Geometry check sheet. Reference: the model listing, model coordinates, mm. Coordinates: 2 decimals unless noted, no trailing zeros. Loops run counter-clockwise (first coordinate to the right, second up) from the corner with the lowest first, then second, coordinate; pieces in that order, holes last.
from build123d import *

# Parameters (mm, degrees)
SKETCH_1_W          = 482.6
SKETCH_1_H          = 88.1
EXTRUDE_1_DEPTH     = 4
CUT_EXTRUDE_1_DEPTH = 491.591856842
SKETCH_3_R          = 3
CUT_EXTRUDE_2_DEPTH = 491.591856842
SKETCH_4_W          = 86
SKETCH_4_H          = 55.5
CUT_EXTRUDE_3_DEPTH = 491.591856842


with BuildPart() as part:
    # Эскиз1 → Бобышка-Вытянуть1 (new body)
    with BuildSketch(Plane.XY):
        with Locations((241.3, 44.05)):
            Rectangle(SKETCH_1_W, SKETCH_1_H)
    extrude(amount=EXTRUDE_1_DEPTH)

    # Эскиз2 → Вырез-Вытянуть1 (cut, through all)
    with BuildSketch(Plane.XY.offset(4)):
        with BuildLine():
            Line((6.8, 76.12), (10.1, 76.12))
            ThreePointArc((10.1, 76.12), (13.6, 72.62), (10.1, 69.12))
            Line((10.1, 69.12), (6.8, 69.12))
            ThreePointArc((6.8, 69.12), (3.3, 72.62), (6.8, 76.12))
        make_face()
        with BuildLine():
            Line((472.5, 76.12), (475.8, 76.12))
            ThreePointArc((475.8, 76.12), (479.3, 72.62), (475.8, 69.12))
            Line((475.8, 69.12), (472.5, 69.12))
            ThreePointArc((472.5, 69.12), (469, 72.62), (472.5, 76.12))
        make_face()
        with BuildLine():
            Line((472.5, 18.97), (475.8, 18.97))
            ThreePointArc((475.8, 18.97), (479.3, 15.47), (475.8, 11.97))
            Line((475.8, 11.97), (472.5, 11.97))
            ThreePointArc((472.5, 11.97), (469, 15.47), (472.5, 18.97))
        make_face()
        with BuildLine():
            Line((6.8, 18.97), (10.1, 18.97))
            ThreePointArc((10.1, 18.97), (13.6, 15.47), (10.1, 11.97))
            Line((10.1, 11.97), (6.8, 11.97))
            ThreePointArc((6.8, 11.97), (3.3, 15.47), (6.8, 18.97))
        make_face()
    extrude(amount=-CUT_EXTRUDE_1_DEPTH, mode=Mode.SUBTRACT)

    # Эскиз3 → Вырез-Вытянуть2 (cut, through all)
    with BuildSketch(Plane.XY.offset(4)):
        with Locations((78.3, 78.1)):
            Circle(SKETCH_3_R)
        with Locations((404.3, 78.1)):
            Circle(SKETCH_3_R)
        with Locations((404.3, 10)):
            Circle(SKETCH_3_R)
        with Locations((78.3, 10)):
            Circle(SKETCH_3_R)
        with Locations((48.3, 78.1)):
            Circle(SKETCH_3_R)
        with Locations((434.3, 78.1)):
            Circle(SKETCH_3_R)
        with Locations((434.3, 10)):
            Circle(SKETCH_3_R)
        with Locations((48.3, 10)):
            Circle(SKETCH_3_R)
    extrude(amount=-CUT_EXTRUDE_2_DEPTH, mode=Mode.SUBTRACT)

    # Эскиз4 → Вырез-Вытянуть3 (cut, through all)
    with BuildSketch(Plane.XY.offset(4)):
        with Locations((145, 45.35)):
            Rectangle(SKETCH_4_W, SKETCH_4_H)
    extrude(amount=-CUT_EXTRUDE_3_DEPTH, mode=Mode.SUBTRACT)


solid = part.part
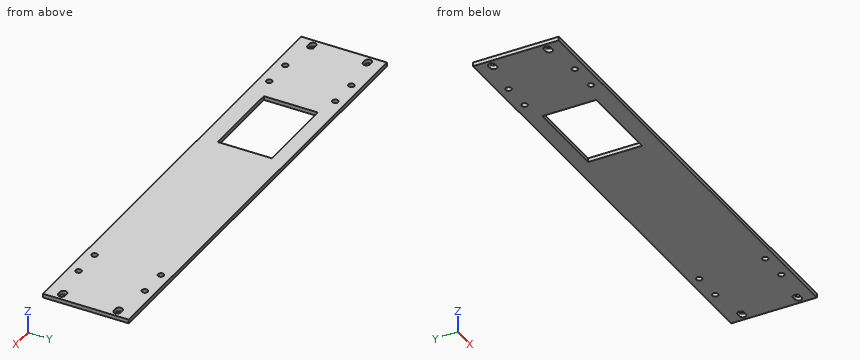
1) Material ranges on probe 1 along Y at (x, z) = (404.3, 2.6); probe 2 along X at (y, z) = (32, 3.7); probe 3 along Y at (x, z) = (138, 2.5), recorded low to high.
Data:
probe 1: y = 0 to 7, 13 to 75.1, 81.1 to 88.1
probe 2: x = 0 to 102, 188 to 482.6
probe 3: y = 0 to 17.6, 73.1 to 88.1
2) Depth check by flat-ended pin: pin 1 (5.5 mm diameter, centred on x = 404.3, y = 10, fed in from -Z). Enter the tip coordinate at first touch or a pass-through.
Data:
pin 1: passes through
3) Section check A-A on x = 137. Record the cut outline in (y, z).
Data:
outline: (0, 0) - (17.6, 0) - (17.6, 4) - (0, 4) - close; (73.1, 0) - (88.1, 0) - (88.1, 4) - (73.1, 4) - close
4) Section check C-C on z = 3. Count the separate pieces of the cut face and the enclosed holes in it, and give its area (3 significant figures).
Data:
separate pieces: 1
enclosed holes: 13
area: 37,300 mm2
5) Section check B-B on y = 36.5. Record the cut outline in (x, z).
Data:
outline: (0, 0) - (102, 0) - (102, 4) - (0, 4) - close; (188, 0) - (482.6, 0) - (482.6, 4) - (188, 4) - close
